For this review, take the finished solid that the model builds, in its own axes (mm). Give positions to 0.01 mm unless a question says otherwise; leave off trailing zeros. Order: outer loops, then holes, each group sorted by start corner. A loop starts at its lowest first (then second) coordinate and runs counter-clockwise, first axis right, second up. Notation, with made-up numbers: (32, 14.5) -> (70, 14.5) arc R21 ccw to (70, 19.5) -> close; hole circle Ø10 at (-3.5, 14). An arc over 180 degrees is marked (long way). One line per item, written item: value. Start each with the question number.
from build123d import *

# Parameters (mm, degrees)
SKETCH1_W           = 88.9
SKETCH1_H           = 228.6
BOSS_EXTRUDE1_DEPTH = 3.175
SKETCH12_R          = 3.3782
SKETCH12_W          = 39.37
SKETCH12_H          = 63.5
CUT_EXTRUDE13_DEPTH = 4.175
SKETCH14_R          = 2.5527
CUT_EXTRUDE15_DEPTH = 4.175
SKETCH15_W          = 88.9
SKETCH15_H          = 57.15
CUT_EXTRUDE16_DEPTH = 4.175
FILLET1_R           = 3.175
SKETCH18_R          = 1.6891
CUT_EXTRUDE18_DEPTH = 4.175
SKETCH16_R          = 3.3782
BOSS_EXTRUDE2_DEPTH = 3.175
SKETCH19_R          = 3.3782
CUT_EXTRUDE19_DEPTH = 4.175
SKETCH20_R          = 1.143
CUT_EXTRUDE20_DEPTH = 4.175
SKETCH21_W          = 88.9
SKETCH21_H          = 3.175
BOSS_EXTRUDE3_DEPTH = 19.05
CUT_EXTRUDE21_DEPTH = 4.175
CUT_EXTRUDE22_DEPTH = 4.175


with BuildPart() as part:
    # Sketch1 → Boss-Extrude1 (new body)
    with BuildSketch(Plane(origin=(0, 0, 0), x_dir=(1, 0, 0), z_dir=(0, 1, 0))):
        Rectangle(SKETCH1_W, SKETCH1_H)
    extrude(amount=BOSS_EXTRUDE1_DEPTH)

    # Sketch12 → Cut-Extrude13 (cut, through all)
    with BuildSketch(Plane(origin=(0, 3.175, 0), x_dir=(1, 0, 0), z_dir=(0, 1, 0))):
        with Locations((29.21, -44.45)):
            Circle(SKETCH12_R)
        with Locations((-29.21, -44.45)):
            Circle(SKETCH12_R)
        with Locations((0, -38.1)):
            Rectangle(SKETCH12_W, SKETCH12_H)
    extrude(amount=-CUT_EXTRUDE13_DEPTH, mode=Mode.SUBTRACT)

    # Sketch14 → Cut-Extrude15 (cut, through all)
    with BuildSketch(Plane(origin=(0, 0, 0), x_dir=(-1, 0, 0), z_dir=(0, -1, 0))):
        with Locations((-37.1475, 107.95)):
            Circle(SKETCH14_R)
        with Locations((-37.1475, 79.883)):
            Circle(SKETCH14_R)
        with Locations((37.1475, 107.95)):
            Circle(SKETCH14_R)
        with Locations((37.1475, 79.883)):
            Circle(SKETCH14_R)
    extrude(amount=-CUT_EXTRUDE15_DEPTH, mode=Mode.SUBTRACT)

    # Sketch15 → Cut-Extrude16 (cut, through all)
    with BuildSketch(Plane.XZ):
        with Locations((0, 85.725)):
            Rectangle(SKETCH15_W, SKETCH15_H)
        with BuildLine():
            Line((12.7, -51.308), (12.7, -17.991666667))
            ThreePointArc((12.7, -17.991666667), (11.77006403, -15.746602636), (9.525, -14.816666667))
            Line((9.525, -14.816666667), (-9.525, -14.816666667))
            ThreePointArc((-9.525, -14.816666667), (-11.77006403, -15.746602636), (-12.7, -17.991666667))
            Line((-12.7, -17.991666667), (-12.7, -51.308))
            ThreePointArc((-12.7, -51.308), (-11.77006403, -53.55306403), (-9.525, -54.483))
            Line((-9.525, -54.483), (9.525, -54.483))
            ThreePointArc((9.525, -54.483), (11.77006403, -53.55306403), (12.7, -51.308))
        make_face()
        with BuildLine():
            Line((12.7, 6.35), (-12.7, 6.35))
            Line((-12.7, 6.35), (-12.7, 1.058333333))
            ThreePointArc((-12.7, 1.058333333), (-11.77006403, -1.186730697), (-9.525, -2.116666667))
            Line((-9.525, -2.116666667), (9.525, -2.116666667))
            ThreePointArc((9.525, -2.116666667), (11.77006403, -1.186730697), (12.7, 1.058333333))
            Line((12.7, 1.058333333), (12.7, 6.35))
        make_face()
    extrude(amount=-CUT_EXTRUDE16_DEPTH, mode=Mode.SUBTRACT)

    # Fillet1
    fillet1_edges = [part.edges().sort_by_distance(p)[0] for p in [
        (19.685, 1.5875, 6.35),
        (-19.685, 1.5875, 6.35),
        (-12.7, 1.5875, 6.35),
        (12.7, 1.5875, 6.35),
    ]]
    fillet(fillet1_edges, radius=FILLET1_R)

    # Sketch18 → Cut-Extrude18 (cut, through all)
    with BuildSketch(Plane(origin=(0, 3.175, 0), x_dir=(1, 0, 0), z_dir=(0, 1, 0))):
        with Locations((-23.9014, 29.083)):
            Circle(SKETCH18_R)
        with Locations((23.9014, 27.98318)):
            Circle(SKETCH18_R)
        with Locations((-8.70204, 79.883)):
            Circle(SKETCH18_R)
        with Locations((19.19986, 79.883)):
            Circle(SKETCH18_R)
    extrude(amount=-CUT_EXTRUDE18_DEPTH, mode=Mode.SUBTRACT)

    # Sketch16 → Boss-Extrude2 (add)
    with BuildSketch(Plane(origin=(0, 3.175, 0), x_dir=(1, 0, 0), z_dir=(0, 1, 0))):
        with BuildLine():
            Line((-44.45, -57.15), (-44.45, -76.2))
            ThreePointArc((-44.45, -76.2), (-32.0675, -88.5825), (-19.685, -76.2))
            Line((-19.685, -76.2), (-19.685, -57.15))
            Line((-19.685, -57.15), (-44.45, -57.15))
        make_face()
        with Locations((-32.0675, -76.2)):
            Circle(SKETCH16_R, mode=Mode.SUBTRACT)
        with BuildLine():
            ThreePointArc((44.45, -76.2), (32.0675, -88.5825), (19.685, -76.2))
            Line((19.685, -76.2), (19.685, -57.15))
            Line((19.685, -57.15), (44.45, -57.15))
            Line((44.45, -57.15), (44.45, -76.2))
        make_face()
        with Locations((32.0675, -76.2)):
            Circle(SKETCH16_R, mode=Mode.SUBTRACT)
    extrude(amount=-BOSS_EXTRUDE2_DEPTH)

    # Sketch19 → Cut-Extrude19 (cut, through all)
    with BuildSketch(Plane(origin=(0, 3.175, 0), x_dir=(1, 0, 0), z_dir=(0, 1, 0))):
        with Locations((-25.4, 60.536666667)):
            Circle(SKETCH19_R)
        with Locations((25.4, 60.536666667)):
            Circle(SKETCH19_R)
    extrude(amount=-CUT_EXTRUDE19_DEPTH, mode=Mode.SUBTRACT)

    # Sketch20 → Cut-Extrude20 (cut, through all)
    with BuildSketch(Plane(origin=(0, 3.175, 0), x_dir=(1, 0, 0), z_dir=(0, 1, 0))):
        with Locations((-32.0675, -26.58657951)):
            Circle(SKETCH20_R)
        with Locations((32.0675, -26.58657951)):
            Circle(SKETCH20_R)
        with BuildLine():
            Line((-25.4635, -24.384), (-38.6715, -24.384))
            ThreePointArc((-38.6715, -24.384), (-40.259, -22.7965), (-38.6715, -21.209))
            Line((-38.6715, -21.209), (-38.6715, -4.191))
            ThreePointArc((-38.6715, -4.191), (-40.259, -2.6035), (-38.6715, -1.016))
            Line((-38.6715, -1.016), (-35.687, -1.016))
            ThreePointArc((-35.687, -1.016), (-34.564467985, -0.551032015), (-34.0995, 0.5715))
            Line((-34.0995, 0.5715), (-34.0995, 0.6985))
            ThreePointArc((-34.0995, 0.6985), (-33.634532015, 1.821032015), (-32.512, 2.286))
            Line((-32.512, 2.286), (-31.623, 2.286))
            ThreePointArc((-31.623, 2.286), (-30.500467985, 1.821032015), (-30.0355, 0.6985))
            Line((-30.0355, 0.6985), (-30.0355, 0.5715))
            ThreePointArc((-30.0355, 0.5715), (-29.570532015, -0.551032015), (-28.448, -1.016))
            Line((-28.448, -1.016), (-25.4635, -1.016))
            ThreePointArc((-25.4635, -1.016), (-23.876, -2.6035), (-25.4635, -4.191))
            Line((-25.4635, -4.191), (-25.4635, -21.209))
            ThreePointArc((-25.4635, -21.209), (-23.876, -22.7965), (-25.4635, -24.384))
        make_face()
        with BuildLine():
            Line((25.4635, -24.384), (38.6715, -24.384))
            ThreePointArc((38.6715, -24.384), (40.259, -22.7965), (38.6715, -21.209))
            Line((38.6715, -21.209), (38.6715, -4.191))
            ThreePointArc((38.6715, -4.191), (40.259, -2.6035), (38.6715, -1.016))
            Line((38.6715, -1.016), (35.687, -1.016))
            ThreePointArc((35.687, -1.016), (34.564467985, -0.551032015), (34.0995, 0.5715))
            Line((34.0995, 0.5715), (34.0995, 0.6985))
            ThreePointArc((34.0995, 0.6985), (33.634532015, 1.821032015), (32.512, 2.286))
            Line((32.512, 2.286), (31.623, 2.286))
            ThreePointArc((31.623, 2.286), (30.500467985, 1.821032015), (30.0355, 0.6985))
            Line((30.0355, 0.6985), (30.0355, 0.5715))
            ThreePointArc((30.0355, 0.5715), (29.570532015, -0.551032015), (28.448, -1.016))
            Line((28.448, -1.016), (25.4635, -1.016))
            ThreePointArc((25.4635, -1.016), (23.876, -2.6035), (25.4635, -4.191))
            Line((25.4635, -4.191), (25.4635, -21.209))
            ThreePointArc((25.4635, -21.209), (23.876, -22.7965), (25.4635, -24.384))
        make_face()
    extrude(amount=-CUT_EXTRUDE20_DEPTH, mode=Mode.SUBTRACT)

    # Sketch21 → Boss-Extrude3 (add)
    with BuildSketch(Plane(origin=(0, 0, -114.3), x_dir=(-1, 0, 0), z_dir=(0, 0, -1))):
        with Locations((0, 1.5875)):
            Rectangle(SKETCH21_W, SKETCH21_H)
    extrude(amount=BOSS_EXTRUDE3_DEPTH)

    # Sketch22 → Cut-Extrude21 (cut, through all)
    with BuildSketch(Plane(origin=(0, 3.175, 0), x_dir=(1, 0, 0), z_dir=(0, 1, 0))):
        with BuildLine():
            Line((-44.45, 133.35), (-31.75, 133.35))
            Line((-31.75, 133.35), (-31.75, 117.475))
            ThreePointArc((-31.75, 117.475), (-32.67993597, 115.22993597), (-34.925, 114.3))
            Line((-34.925, 114.3), (-44.45, 114.3))
            Line((-44.45, 114.3), (-44.45, 133.35))
        make_face()
        with BuildLine():
            Line((44.45, 114.3), (34.925, 114.3))
            ThreePointArc((34.925, 114.3), (32.67993597, 115.22993597), (31.75, 117.475))
            Line((31.75, 117.475), (31.75, 133.35))
            Line((31.75, 133.35), (44.45, 133.35))
            Line((44.45, 133.35), (44.45, 114.3))
        make_face()
    extrude(amount=-CUT_EXTRUDE21_DEPTH, mode=Mode.SUBTRACT)

    # Sketch23 → Cut-Extrude22 (cut, through all)
    with BuildSketch(Plane(origin=(0, 3.175, 0), x_dir=(1, 0, 0), z_dir=(0, 1, 0))):
        with BuildLine():
            Line((-38.25875, -63.777875899), (-38.25875, -36.901440438))
            ThreePointArc((-38.25875, -36.901440438), (-39.18868597, -34.656376407), (-41.43375, -33.726440438))
            Line((-41.43375, -33.726440438), (-44.45, -33.726440438))
            Line((-44.45, -33.726440438), (-44.45, -76.2))
            ThreePointArc((-44.45, -76.2), (-43.149805735, -70.676522306), (-39.522270408, -66.313003266))
            ThreePointArc((-39.522270408, -66.313003266), (-38.592133145, -65.194152231), (-38.25875, -63.777875899))
        make_face()
        with BuildLine():
            Line((41.43375, -33.726440438), (44.45, -33.726440438))
            Line((44.45, -33.726440438), (44.45, -76.2))
            ThreePointArc((44.45, -76.2), (43.149805735, -70.676522306), (39.522270408, -66.313003266))
            ThreePointArc((39.522270408, -66.313003266), (38.592133145, -65.194152231), (38.25875, -63.777875899))
            Line((38.25875, -63.777875899), (38.25875, -36.901440438))
            ThreePointArc((38.25875, -36.901440438), (39.18868597, -34.656376407), (41.43375, -33.726440438))
        make_face()
    extrude(amount=-CUT_EXTRUDE22_DEPTH, mode=Mode.SUBTRACT)


solid = part.part
Q1. For line 1 along Z through (x, y) = (-9, 2.15); line 2 along X through (y, z) = (1.05, 44.45) (3 decimals); line 3 along X through (y, z) = (1.8, -60), list the stretches that pass through material, from the lowest coordinate up.
Q2. Mouldability with a two-part tool opening along X and no side actions: class faces 1 (the cylindrical face through (-35.27, 1.57, -109.68)), 2 (the flat face through (20, 3.175, -45)), 3 (the cylindrical face through (22.91, 1.61, -62.82)) as pulls with the +X half, pulls with the -X half, needs draft (parallel to the pull), parting line crosses it, or undercut.
Q3. Take a section at B-B (x = 4.5). State the section outline as (y, z) points (3 decimals), and give its area (3 significant figures).
Q4. Take a section at A-A (z = 44.45). State the section outline as (x, y) points (3 decimals).
Q5. For pin 1 Ø4 at (x, z) = (-29.21, 44.45) entering from +Y; pin 2 Ø0.5 at (x, y) = (16, 1.5) entering from +Z; pin 3 Ø5.5 at (x, z) = (19.2, -79.88) entering from +Y (3 decimals); pin 4 Ø1 at (x, y) = (-1, 2.5) entering from +Z, all flat-tipped, find the tip position at first contact; note any pin that passes through.
Q6. Take a section at C-C (z = -107.95). State the section outline as (x, y) points (3 decimals).
Q7. Take a section at D-D (y = 1). State how many separate pieces and enclosed holes the cut face has, and give its area (3 significant figures).
Answers below:
1. line 1: z = -133.35 to -81.55, -78.22 to -54.48, -14.82 to -2.12
1. line 2: x = -38.259 to -32.588, -25.832 to -19.685, 19.685 to 25.832, 32.588 to 38.259
1. line 3: x = -44.45 to -28.74, -22.06 to 22.06, 28.74 to 44.45
2. face 1: undercut
2. face 2: needs draft
2. face 3: undercut
3. outline: (0, -133.35) -> (3.175, -133.35) -> (3.175, -54.483) -> (0, -54.483) -> close; (0, -14.817) -> (3.175, -14.817) -> (3.175, -2.117) -> (0, -2.117) -> close
3. area: 291 mm²
4. outline: (-38.259, 0) -> (-32.588, 0) -> (-32.588, 3.175) -> (-38.259, 3.175) -> close; (-25.832, 0) -> (-19.685, 0) -> (-19.685, 3.175) -> (-25.832, 3.175) -> close; (19.685, 0) -> (25.832, 0) -> (25.832, 3.175) -> (19.685, 3.175) -> close; (32.588, 0) -> (38.259, 0) -> (38.259, 3.175) -> (32.588, 3.175) -> close
5. pin 1: passes through
5. pin 2: stops at z = 6.35
5. pin 3: stops at y = 3.175
5. pin 4: stops at z = -2.12
6. outline: (-44.45, 0) -> (-39.7, 0) -> (-39.7, 3.175) -> (-44.45, 3.175) -> close; (-34.595, 0) -> (34.595, 0) -> (34.595, 3.175) -> (-34.595, 3.175) -> close; (39.7, 0) -> (44.45, 0) -> (44.45, 3.175) -> (39.7, 3.175) -> close
7. separate pieces: 1
7. enclosed holes: 19
7. area: 13,200 mm²
